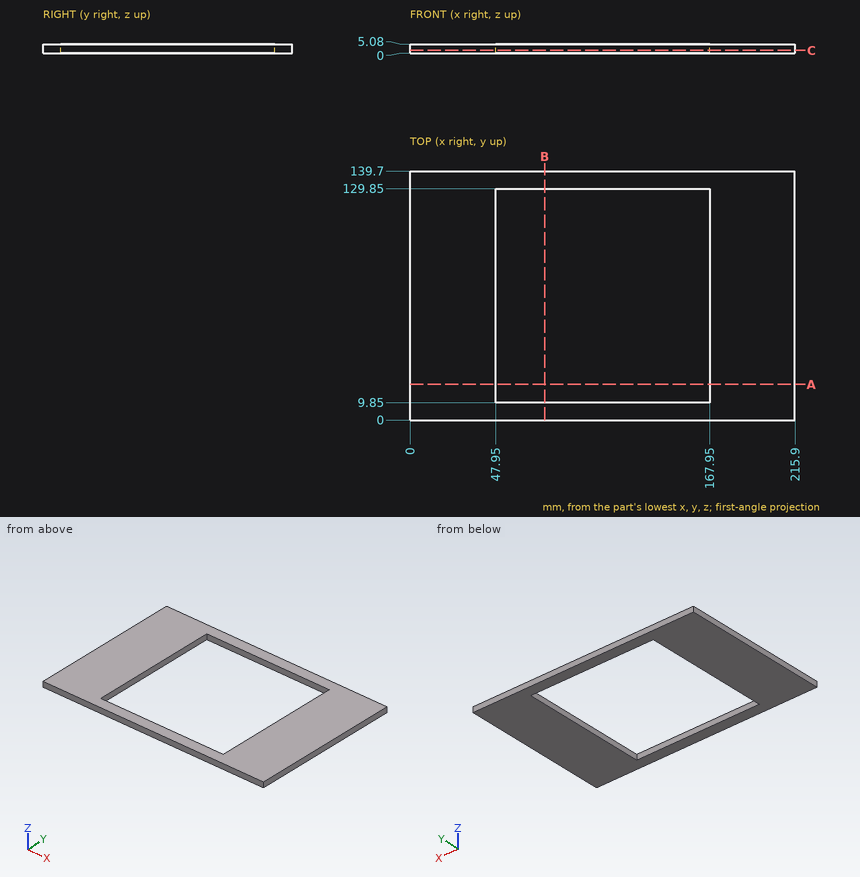
Geometry check sheet. Reference: drawing and pictorial views, mm from the part's lowest x, y, z. Give positions to 0.01 mm unless a question says otherwise; leave off trailing zeros. Order: outer loops, then holes, each group sorted by start corner. A loop starts at its lowest first (then second) coordinate and runs counter-clockwise, first axis right, second up.
1. Section check C-C, the plane z = 1.55. Enter the section's corners in (x, y), and give its area (3 significant figures).
2. Section check A-A, the plane y = 20. Enter the section's corners in (x, z), and give its area (3 significant figures).
3. Thickness scan on L1, parallel to X at y = 102, z = 2.5; L2, parallel to Y at x = 161.5, z = 4. Record the ranges inside material, lowest first.
4. Section check B-B, the plane x = 75.5. Enter the section's corners in (y, z), and give its area (3 significant figures).
Values follow:
1. outline: (0, 0) - (215.9, 0) - (215.9, 139.7) - (0, 139.7) - close; hole (47.95, 9.85) - (167.95, 9.85) - (167.95, 129.85) - (47.95, 129.85) - close
1. area: 15,800 mm2
2. outline: (0, 0) - (47.95, 0) - (47.95, 5.08) - (0, 5.08) - close; (167.95, 0) - (215.9, 0) - (215.9, 5.08) - (167.95, 5.08) - close
2. area: 487 mm2
3. L1: x = 0 to 47.95, 167.95 to 215.9
3. L2: y = 0 to 9.85, 129.85 to 139.7
4. outline: (0, 0) - (9.85, 0) - (9.85, 5.08) - (0, 5.08) - close; (129.85, 0) - (139.7, 0) - (139.7, 5.08) - (129.85, 5.08) - close
4. area: 100 mm2
